Answer from the drawing. Dimensions are ordinates in mm from the lowest x, y and z of the part. A direction names the side the tool comes from. Coordinates: 2 decimals unless noted, no trailing zeros. Order: outer loops, then holes, each group sorted by start corner. A loop starts at its lowest first (then second) coordinate and runs counter-clockwise, first axis right, second up. Notation, with made-up numbers: M 36,28.25 L 63,28.25 A33 cw 63,63.25 Z; hole C -10.75,79.5 d6. An arc over 180 degrees is marked long. One line per question, with ' | ' between items. Start each with the question number.
1) Consider probe 1 along X at (y, z) = (1, 2.5); probe 2 along X at (y, z) = (0.7, 53.3); probe 3 along Z at (x, y) = (18.2, 0.55). Determine where each line is inside the solid, lowest interval first.
2) A tool of negligible diameter and unlimited length cuts with its end or side. For the marked faces 5, 6, 7 and 8, from which of +Z, -Z, +X, -X, +Y, -Y can it reach the whole face along a straight path? Write none if from no direction.
3) Find section C-C, the plane x = 18.2. Write down the section's boundary in (y, z) (3 decimals).
4) Find section D-D, the plane z = 46.5. Write down the section's boundary in (x, y).
5) Given P1, Ø3, axis at x = 16.5, y = 7, coming from the -Z side (3 decimals); P2, Ø5.5, axis at y = 8, z = 63, coming from the -X side (3 decimals); P3, Ø3, axis at x = 44, z = 72, coming from the -Y side; P4, Ø5, axis at x = 6, y = 9, coming from the +Z side, each flat-ended and moving along its own axis, determine where each tip first touches the part or whether it passes through.
6) The mould has two halves that part along X. Classify the marked faces 1, 2, 3 and 4: +X half, -X half, draft (parallel to the pull), parting line (faces both ways), or undercut.
7) Find section B-B, the plane y = 9.5. Write down the section's boundary in (x, z) (3 decimals).
8) Find section A-A, the plane x = 50.8. Write down the section's boundary in (y, z).
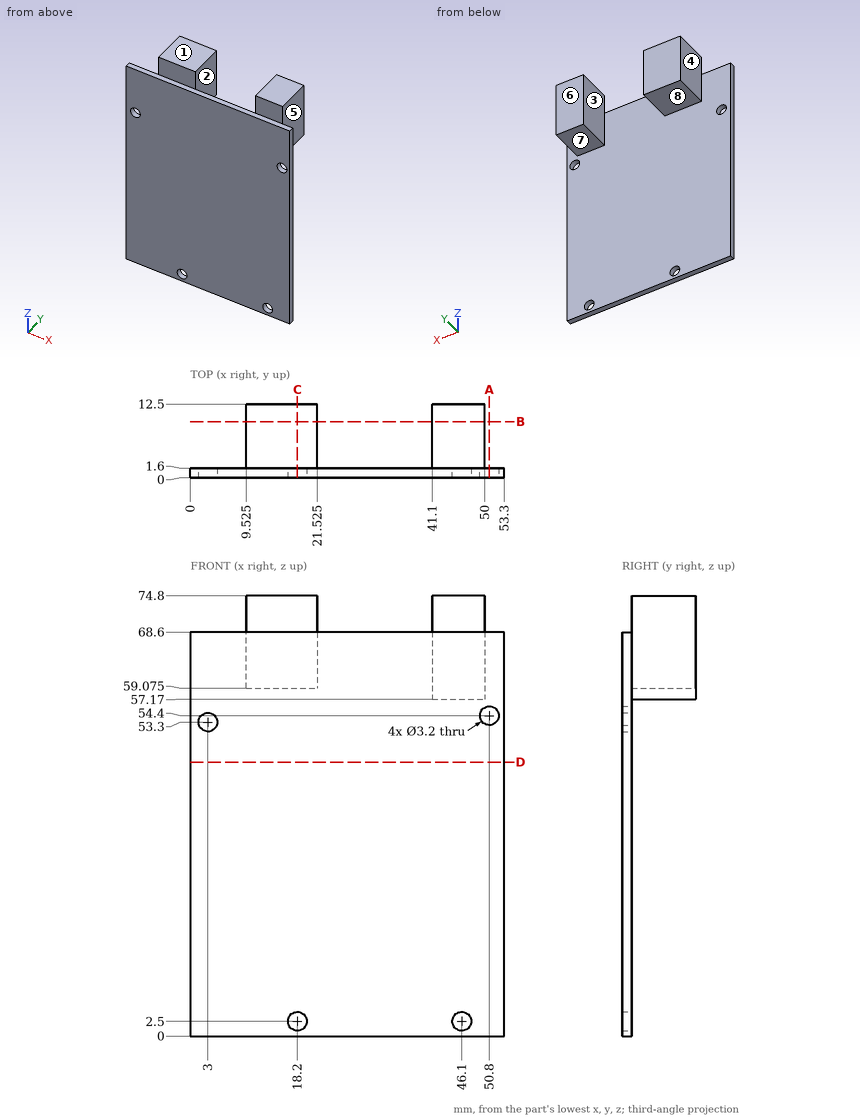
Report:
1) probe 1: x = 0 to 16.6, 19.8 to 44.5, 47.7 to 53.3 | probe 2: x = 0 to 1.4, 4.6 to 49.64, 51.96 to 53.3 | probe 3: z = 0 to 0.9, 4.1 to 68.6
2) face 5: +Z, -Z, +X, +Y | face 6: +Z, -Z, +X, -X, +Y | face 7: -Z, +X, -X, +Y | face 8: -Z, -X, +Y
3) outline: M 0,0 L 1.6,0 L 1.6,0.9 L 0,0.9 Z; M 0,4.1 L 1.6,4.1 L 1.6,59.075 L 12.5,59.075 L 12.5,74.8 L 1.6,74.8 L 1.6,68.6 L 0,68.6 Z
4) outline: M 0,0 L 53.3,0 L 53.3,1.6 L 0,1.6 Z
5) P1: stops at z = 59.075 | P2: stops at x = 9.525 | P3: stops at y = 1.6 | P4: passes through
6) face 1: draft | face 2: undercut | face 3: undercut | face 4: -X half
7) outline: M 9.525,59.075 L 21.525,59.075 L 21.525,74.8 L 9.525,74.8 Z; M 41.1,57.17 L 50,57.17 L 50,74.8 L 41.1,74.8 Z
8) outline: M 0,0 L 1.6,0 L 1.6,52.8 L 0,52.8 Z; M 0,56 L 1.6,56 L 1.6,68.6 L 0,68.6 Z
